CAD build for the part. Positions are in the model's coordinates, mm. A direction names the side the tool comes from. Round coordinates to 2 decimals unless told otherwise and drop trailing zeros. Order: outer loops, then holes, each group sorted by start corner. A loop starts at its lowest first (then second) coordinate and runs counter-clockwise, first axis right, second up. Notation, with made-up numbers: M 82.5,38.25 L 110.5,38.25 A18 ccw 110.5,73.25 Z; hole C 47,77 d8. An arc over 180 degrees is marked long. Put each result on its own line as item: value.
```python
from build123d import *

# Parameters (mm, degrees)
F0_W     = 90
F0_H     = 374.65
F2_R     = 30
F3_DEPTH = 374.651
F4_R     = 36.5
F4_R_2   = 30
F5_DEPTH = 346


with BuildPart() as f1:
    # F0 (on Front) → F1 (revolve)
    with BuildSketch(Plane.XZ):
        with Locations((45, -187.325)):
            Rectangle(F0_W, F0_H)
    revolve(axis=Axis((0, 0, -187.325), (0, 0, -1)))

    # F2 (on face) → F3 (cut, through all)
    with BuildSketch(Plane.XY):
        with Locations((0, 2.491364)):
            Circle(F2_R)
    extrude(amount=-F3_DEPTH, mode=Mode.SUBTRACT)

    # F4 (on face) → F5 (cut)
    with BuildSketch(Plane.XY):
        Circle(F4_R)
        with Locations((0, 2.491364)):
            Circle(F4_R_2, mode=Mode.SUBTRACT)
    extrude(amount=-F5_DEPTH, mode=Mode.SUBTRACT)


solid = f1.part
```
Item 1: Band-saw the part on B-B on z = -214. Give the cut face in (x, y), and give its area (3 significant figures).
Answers below:
outline: C 0,0 d180; hole C 0,0 d73
area: 21,300 mm²
Item 2: Probe line 1 along Y through (x, z) = (0, -352); line 2 along Y through (x, z) = (0, -137); line 3 along X through (y, z) = (-14.5, -238). List the from-to ranges inside material, lowest first. Write a range as [from, to].
Answers below:
line 1: [-90, -27.51], [32.49, 90]
line 2: [-90, -36.5], [36.5, 90]
line 3: [-88.82, -33.5], [33.5, 88.82]
Item 3: Pin check, flat tips, straight feed: P1, Ø1.5, axis at x = -30.5, z = -118, coming from the +Y side; P2, Ø1.5, axis at y = 24, z = -80.5, coming from the +X side (3 decimals); P3, Ø5, axis at x = -63, y = 69, coming from the -Z side; P4, Ø10, axis at y = 61, z = -41.5, coming from the -X side. Stop position of each tip, or through.
Answers below:
P1: y = 84.94
P2: x = 86.945
P3: through
P4: x = -70.46
Item 4: Band-saw the part on C-C on y = 57. Give the cut face in (x, z).
Answers below:
outline: M -69.65,-374.65 L 69.65,-374.65 L 69.65,0 L -69.65,0 Z
Item 5: Band-saw the part on D-D on x = -65. Give the cut face in (y, z).
Answers below:
outline: M -62.25,-374.65 L 62.25,-374.65 L 62.25,0 L -62.25,0 Z
Item 6: Mould opens along X. For faces 3 (the cylindrical face through (41.53, 79.845, -184.702)), 4 (the flat face through (-11, -27, -346)), 5 (the flat face through (1, 39, 0)) say: pulls with the +X half, pulls with the -X half, needs draft (parallel to the pull), parting line crosses it, or undercut.
Answers below:
face 3: parting line crosses it
face 4: undercut
face 5: needs draft
Item 7: Tool access for faces 1 (the cylindrical face through (-7.912, -35.632, -170.578)), 2 (the flat face through (-19, -21, -374.65)): list every direction of +Z, -Z, +X, -X, +Y, -Y with a clear straight run to the whole face (end or side of a thin tool).
Answers below:
face 1: +Z
face 2: -Z, +X, -X, +Y, -Y
Item 8: Band-saw the part on A-A on x = 0. Give the cut face in (y, z), and give its area (3 significant figures).
Answers below:
outline: M -90,-374.65 L -27.51,-374.65 L -27.51,-346 L -36.5,-346 L -36.5,0 L -90,0 Z; M 32.49,-374.65 L 90,-374.65 L 90,0 L 36.5,0 L 36.5,-346 L 32.49,-346 Z
area: 40,500 mm²
